The listing builds one solid part. Answer for the finished solid, in the listing's coordinates (mm). Face numbers are marked on the shaded views. A direction names the side the tool comes from. Round coordinates to 2 decimals unless told otherwise and drop trailing zeros. Loops run counter-clockwise (first coordinate to the right, second up) from the corner with the lowest first, then second, coordinate; pieces in that order, holes last. Notation, with made-up numbers: (28, 0.25) -> (82, 0.25) arc R19 cw to (82, 31.25) -> close; hole circle Ø3 at (26, 2.5). An arc over 180 degrees is marked (long way). Use a Markdown table: item, result. Add a question column.
Q1. Section B-B on x = 0 is taken. Give the vertices of the cut face in (y, z).
Q2. For a pull along Z with two mould halves and no side action, classify the marked faces 1, 2 and 3 as released by +Z, released by -Z, zero draft, split by the parting line, or undercut.
Q3. Section C-C on z = 25.5 is taken. Give the vertices of the cut face in (x, y).
Q4. Consider line 1 (Y direction, x = -11.5, z = 103); line 2 (X direction, y = 89, z = 137.5); line 3 (Z direction, x = -46.5, y = 63). Determine where each line is inside the solid, lowest interval first.
Q5. Section A-A on y = 27 is taken. Give the vertices of the cut face in (x, z).
Q6. Which of the six approach directions +Z, -Z, +X, -X, +Y, -Y give full straight-line access (tool end or side, diameter ignored) to the marked faces 4 and 5?
Q7. Section D-D on y = 45.5 is taken. Give the vertices of the cut face in (x, z).
Q8. Given pin 1 Ø10 at (y, z) = (88.5, 44.5) entering from +X; pin 2 Ø11 at (x, z) = (-92, 8) entering from +Y; pin 3 Ø11 at (x, z) = (1, 86) entering from -Y, each flat-ended and moving along its own axis, determine where each tip first touches the part or whether it passes through.
from build123d import *

# Parameters (mm, degrees)
F1_DEPTH    = 15
F2_W        = 32
F2_H        = 23
F3_DEPTH    = 150
F4_T        = 2.5
F4_T3_DEPTH = 28
F4_T5_DEPTH = 37
F5_R        = 5


# Not quite as in the source:
# - a shell that OpenCascade refuses in one call is made with other operations: the cavity is built on its own and cut out


with BuildPart() as f1:
    # F0 (on Top) → F1 (new body)
    with BuildSketch(Plane.XY):
        with BuildLine():
            Line((75, 0), (100, 0))
            ThreePointArc((100, 0), (0, 100), (-100, 0))
            Line((-100, 0), (-75, 0))
            ThreePointArc((-75, 0), (0, 75), (75, 0))
        make_face()
    extrude(amount=F1_DEPTH)

    # F2 (on face) → F3 (join)
    with BuildSketch(Plane.XY.offset(15)):
        with Locations((0, 87.211701434)):
            Rectangle(F2_W, F2_H)
    extrude(amount=F3_DEPTH)

    # F4: shell of thickness 2.5, made by hand


with BuildPart() as f4_core1:
    # F4_t2: copy of F1
    add(f1.part)

    # the walls: a layer under each face that stays
    f4_faces = [f4_core1.faces().sort_by_distance(p)[0] for p in [
        (-87.5, 0, 7.5),
        (0, 100, 7.5),
        (0, 75, 7.5),
        (-66.6666666667, 50, 0),
        (-66.6666666667, 49.355850717, 15),
        (87.5, 0, 7.5),
        (0, 99.355850717, 15),
        (-16, 87.211701434, 90),
        (0, 75.711701434, 90),
        (16, 87.211701434, 90),
        (0, 98.711701434, 90),
    ]]
    thicken(f4_faces, amount=-F4_T, mode=Mode.SUBTRACT)

    # F4_s4 → F4_t3 (cut)
    with BuildSketch(Plane.XZ.offset(-101.211701434)):
        Polygon((-16.025, 15.025), (-16, 12.5), (-13.5, 12.5), (-13.5, 15), align=None)
        Polygon((16.025, 15.025), (16, 12.5), (13.5, 12.5), (13.5, 15), align=None)
    extrude(amount=F4_T3_DEPTH, mode=Mode.SUBTRACT)

    # F4_s6 → F4_t5 (cut)
    with BuildSketch(Plane.YZ.offset(-18.5)):
        Polygon((75.686701434, 15.025), (75.711701434, 12.5), (78.211701434, 12.5), (78.211701434, 15), align=None)
        Polygon((98.736701434, 15.025), (98.711701434, 12.5), (96.211701434, 12.5), (96.211701434, 15), align=None)
    extrude(amount=F4_T5_DEPTH, mode=Mode.SUBTRACT)


with BuildPart() as f1_1:
    add(f1.part)

    # what is left inside the walls is the cavity
    f4_cavity = [f4_core1.part.solids().sort_by_distance(p)[0] for p in [
        (-48.733972, 65.833333, 2.525),
    ]]
    add(f4_cavity, mode=Mode.SUBTRACT)

    # F5
    f5_edges = [f1_1.edges().sort_by_distance(p)[0] for p in [
        (-16, 75.711701, 90),
        (-16, 98.711701, 90),
        (16, 98.711701, 90),
        (16, 75.711701, 90),
        (-87.5, 0, 15),
        (-87.5, 0, 0),
        (87.5, 0, 15),
        (87.5, 0, 0),
    ]]
    fillet(f5_edges, radius=F5_R)


solid = f1_1.part
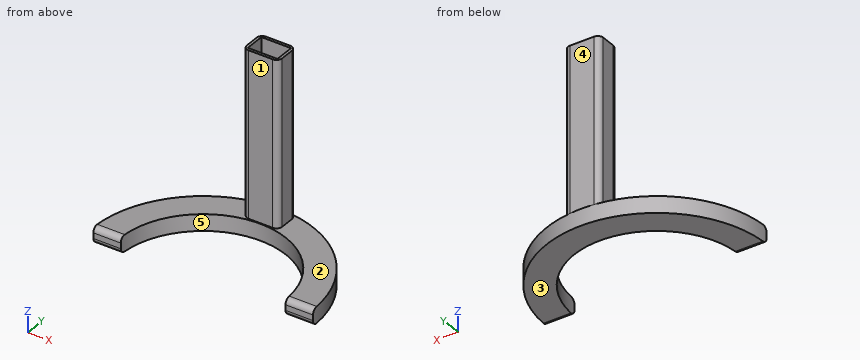
Checked values:
| question | item | result |
|---|---|---|
| 1 | outline | (75, 0) -> (100, 0) -> (100, 15) -> (98.71, 15) -> (98.71, 165) -> (96.21, 165) -> (96.21, 12.5) -> (97.5, 12.5) -> (97.5, 2.5) -> (77.5, 2.5) -> (77.5, 12.5) -> (78.21, 12.5) -> (78.21, 165) -> (75.71, 165) -> (75.71, 15) -> (75, 15) -> close |
| 2 | face 1 | zero draft |
| 2 | face 2 | released by +Z |
| 2 | face 3 | released by -Z |
| 3 | outline | (-16, 80.71) arc R5 ccw to (-11, 75.71) -> (11, 75.71) arc R5 ccw to (16, 80.71) -> (16, 93.71) arc R5 ccw to (11, 98.71) -> (-11, 98.71) arc R5 ccw to (-16, 93.71) -> close; hole (-13.5, 78.21) -> (13.5, 78.21) -> (13.5, 96.21) -> (-13.5, 96.21) -> close |
| 4 | line 1 | y = 75.74 to 78.21, 96.21 to 98.69 |
| 4 | line 2 | x = -16 to -13.5, 13.5 to 16 |
| 4 | line 3 | z = 0 to 2.5, 12.5 to 15 |
| 5 | outline | (-96.29, 0) -> (-69.97, 0) -> (-69.97, 15) -> (-96.29, 15) -> close; (69.97, 0) -> (96.29, 0) -> (96.29, 15) -> (69.97, 15) -> close; hole (-93.69, 2.5) -> (-72.64, 2.5) -> (-72.64, 12.5) -> (-93.69, 12.5) -> close; hole (72.64, 2.5) -> (93.69, 2.5) -> (93.69, 12.5) -> (72.64, 12.5) -> close |
| 6 | face 4 | +Z, +X, -X, +Y |
| 6 | face 5 | +Z, -Z, -Y |
| 7 | outline | (-89.05, 0) -> (-59.62, 0) -> (-59.62, 15) -> (-89.05, 15) -> close; (59.62, 0) -> (89.05, 0) -> (89.05, 15) -> (59.62, 15) -> close; hole (-86.23, 2.5) -> (-62.74, 2.5) -> (-62.74, 12.5) -> (-86.23, 12.5) -> close; hole (62.74, 2.5) -> (86.23, 2.5) -> (86.23, 12.5) -> (62.74, 12.5) -> close |
| 8 | pin 1 | stops at x = 16 |
| 8 | pin 2 | stops at y = 50.18 |
| 8 | pin 3 | stops at y = 75.71 |
